from build123d import *

# Parameters (mm, degrees)
F0_W     = 38.55
F0_H     = 32.85
F1_DEPTH = 0.9
F3_D     = 3.25
F4_W     = 2
F4_H     = 4
F4_W_2   = 4
F4_H_2   = 2
F5_DEPTH = 0.2


with BuildPart() as f1:
    # F0 (on Top) → F1 (new body)
    with BuildSketch(Plane.XY):
        with Locations((0.870858, 0)):
            Rectangle(F0_W, F0_H)
    extrude(amount=F1_DEPTH)

    # F3 (through all)
    with Locations(Plane.XY.offset(0.9)):
        with Locations((-8.879142, 13.05), (8.879142, 13.05), (8.879142, -13.05), (-8.879142, -13.05)):
            Hole(F3_D / 2)

    # F4 (on face) → F5 (cut)
    with BuildSketch(Plane.XY.offset(0.9)):
        with Locations((-2.504142, 14.425)):
            Rectangle(F4_W, F4_H)
        with Locations((3.445858, 14.425)):
            Rectangle(F4_W, F4_H)
        with Locations((18.145858, -2.975)):
            Rectangle(F4_W_2, F4_H_2)
        with Locations((18.145858, -8.425)):
            Rectangle(F4_W_2, F4_H_2)
        with Locations((-16.404142, -8.425)):
            Rectangle(F4_W_2, F4_H_2)
        with Locations((-16.404142, -2.975)):
            Rectangle(F4_W_2, F4_H_2)
    extrude(amount=-F5_DEPTH, mode=Mode.SUBTRACT)


solid = f1.part
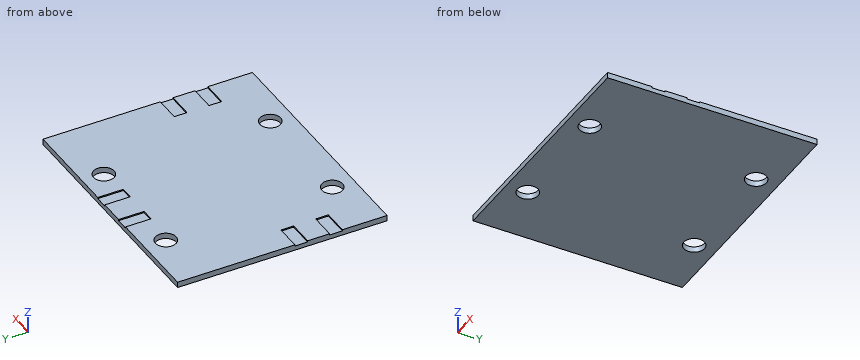
For this review, take the finished solid that the model builds, in its own axes (mm). Round coordinates to 2 decimals unless told otherwise and drop trailing zeros. Loops run counter-clockwise (first coordinate to the right, second up) from the corner with the lowest first, then second, coordinate; pieces in that order, holes last. Notation, with made-up numbers: (70.5, 9.5) - (126.5, 9.5) arc R5 cw to (126.5, 16.5) - close; hole circle Ø3 at (74.25, 61). An arc over 180 degrees is marked (long way). Put each result on its own line as item: value. Start each with the question number.
1. Insertion check: P1, Ø3, axis at x = 8.88, y = -13.05, coming from the +Z side; P2, Ø0.6, axis at x = 18.5, y = -3, coming from the +Z side. Each pin has a flat end and moves straight along its axis. Give the tip position at first contact, or say it passes through.
2. For probe 1 along Y at (x, z) = (7.5, 0.4) (3 decimals); probe 2 along X at (y, z) = (12.5, 0.85); probe 3 along Y at (x, z) = (-8.5, 0.55) (3 decimals), list the stretches that pass through material, from the lowest coordinate up. Write a range as [from, to].
3. Consider section B-B on z = 0.4. State the section outline as (x, y) points (3 decimals).
4. Consider section D-D on y = -13.05. State the section outline as (x, z) points.
5. Consider section C-C on y = -3. State the section outline as (x, z) points.
6. Consider section A-A on y = 13.05. State the section outline as (x, z) points.
Result sheet:
1. P1: through
1. P2: z = 0.7
2. probe 1: [-16.425, -13.909], [-12.191, 12.191], [13.909, 16.425]
2. probe 2: [-18.4, -10.41], [-7.35, -3.5], [-1.5, 2.45], [4.45, 7.35], [10.41, 20.15]
2. probe 3: [-16.425, -14.63], [-11.47, 11.47], [14.63, 16.425]
3. outline: (-18.404, -16.425) - (20.146, -16.425) - (20.146, 16.425) - (-18.404, 16.425) - close; hole circle Ø3.25 at (-8.879, -13.05); hole circle Ø3.25 at (-8.879, 13.05); hole circle Ø3.25 at (8.879, -13.05); hole circle Ø3.25 at (8.879, 13.05)
4. outline: (-18.4, 0) - (-10.5, 0) - (-10.5, 0.9) - (-18.4, 0.9) - close; (-7.25, 0) - (7.25, 0) - (7.25, 0.9) - (-7.25, 0.9) - close; (10.5, 0) - (20.15, 0) - (20.15, 0.9) - (10.5, 0.9) - close
5. outline: (-18.4, 0) - (20.15, 0) - (20.15, 0.7) - (16.15, 0.7) - (16.15, 0.9) - (-14.4, 0.9) - (-14.4, 0.7) - (-18.4, 0.7) - close
6. outline: (-18.4, 0) - (-10.5, 0) - (-10.5, 0.9) - (-18.4, 0.9) - close; (-7.25, 0) - (7.25, 0) - (7.25, 0.9) - (4.45, 0.9) - (4.45, 0.7) - (2.45, 0.7) - (2.45, 0.9) - (-1.5, 0.9) - (-1.5, 0.7) - (-3.5, 0.7) - (-3.5, 0.9) - (-7.25, 0.9) - close; (10.5, 0) - (20.15, 0) - (20.15, 0.9) - (10.5, 0.9) - close
